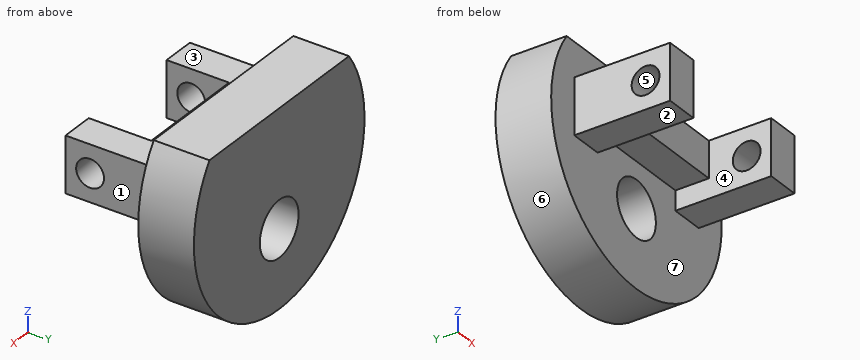
from build123d import *

# Parameters (mm, degrees)
F1_DEPTH = 6.35
F3_D     = 6.35
F2_W     = 3.81
F2_H     = 6.35
F4_DEPTH = 10.9299502
F6_D     = 3.175
F7_W     = 12.7500126
F7_H     = 4.1250048568
F8_DEPTH = 3.81


# Not quite as in the source:
# - a feature names something its author has since deleted; it is built from what else it names


with BuildPart() as f1:
    # F0 (on Front) → F1 (new body)
    with BuildSketch(Plane.XZ):
        with BuildLine():
            Line((11.43, 8.0321852568), (-11.43, 8.0321852568))
            ThreePointArc((-11.43, 8.0321852568), (0, -13.97), (11.43, 8.0321852568))
        make_face()
    extrude(amount=F1_DEPTH)

    # F3 (through all)
    with Locations(Plane.XZ.offset(6.35)):
        with Locations((0, -5.1758147432)):
            Hole(F3_D / 2)

    # F2 (on face) → F4 (join)
    with BuildSketch(Plane.XZ.offset(6.35)):
        with Locations((-8.2800063, 0.9500048568)):
            Rectangle(F2_W, F2_H)
        with Locations((8.2800063, 0.9500048568)):
            Rectangle(F2_W, F2_H)
    extrude(amount=F4_DEPTH)

    # F6 (through all)
    with Locations(Plane(origin=(-10.1850063, 0, 0), x_dir=(0, -1, 0), z_dir=(-1, 0, 0))):
        with Locations((14.478, 0.9500048568)):
            Hole(F6_D / 2)

    # F7 (on face) → F8 (join)
    with BuildSketch(Plane.XZ.offset(6.35)):
        with Locations((0, 2.0625024284)):
            Rectangle(F7_W, F7_H)
    extrude(amount=F8_DEPTH)


solid = f1.part
Part model, mm, in its own coordinate system. Face numbers are marked on the shaded views. A direction names the side the tool comes from. Coordinates: 2 decimals unless noted, no trailing zeros. Loops run counter-clockwise (first coordinate to the right, second up) from the corner with the lowest first, then second, coordinate; pieces in that order, holes last. Notation, with made-up numbers: (-12.5, 18) -> (32.5, 18) arc R22 cw to (32.5, 24) -> close; hole circle Ø10 at (34.25, 19). An arc over 180 degrees is marked (long way). Use a Markdown table: item, result. Add a question column.
Item 1: Band-saw the part on C-C on y = -7.75. Write the cut outline in (x, z) (3 decimals).
Item 2: Probe probe 1 along X at (y, z) = (-14.5, 2.75) (3 decimals); probe 2 along Z at (x, y) = (7.5, -14.5) (3 decimals); probe 3 along Y at (x, z) = (-3, -10.25). List the from-to ranges inside material, lowest first.
Item 3: Flat gauge pins, fed straight in: P1, Ø2, axis at x = -9, y = -3.5, coming from the -Z side; P2, Ø1.9, axis at y = -10, z = 1, coming from the +X side (3 decimals); P3, Ø4, axis at y = -14.48, z = 0.95, coming from the -X side (3 decimals); P4, Ø3.5, axis at x = -3.5, y = -12, coming from the +Z side. Where does each tip first touch, or does it go through?
Item 4: Band-saw the part on B-B on y = -11.75. Write the cut outline in (x, z) (3 decimals).
Item 5: Pull direction Z, two halves, no side cores. Call the marked faces 5, 6 and 7: +Z half, -Z half, draft (parallel to the pull), parting line (faces both ways), or undercut.
Item 6: Which spindle directions (+Z, -Z, +X, -X, +Y, -Y) get a long thin tool onto all of the face, cutting with end or side? Do the marked faces 1, 2, 3 and 4. Say none if no direction does.
Item 7: Band-saw the part on A-A on x = 0. Write the cut outline in (y, z) (3 decimals).
Geometry says:
| question | item | result |
|---|---|---|
| 1 | outline | (-10.185, -2.225) -> (-6.375, -2.225) -> (-6.375, 0) -> (6.375, 0) -> (6.375, -2.225) -> (10.185, -2.225) -> (10.185, 4.125) -> (-10.185, 4.125) -> close |
| 2 | probe 1 | -10.185 to -6.375, 6.375 to 10.185 |
| 2 | probe 2 | -2.225 to -0.637, 2.537 to 4.125 |
| 2 | probe 3 | -6.35 to 0 |
| 3 | P1 | z = -11.45 |
| 3 | P2 | x = 10.185 |
| 3 | P3 | x = -10.185 |
| 3 | P4 | through |
| 4 | outline | (-10.185, -2.225) -> (-6.375, -2.225) -> (-6.375, 4.125) -> (-10.185, 4.125) -> close; (6.375, -2.225) -> (10.185, -2.225) -> (10.185, 4.125) -> (6.375, 4.125) -> close |
| 5 | face 5 | undercut |
| 5 | face 6 | parting line |
| 5 | face 7 | draft |
| 6 | face 1 | +Z, -Z, +X, -Y |
| 6 | face 2 | -Z, +X, -X, -Y |
| 6 | face 3 | +Z, +X, -X, -Y |
| 6 | face 4 | -Z, -Y |
| 7 | outline | (-10.16, 0) -> (-6.35, 0) -> (-6.35, -2.001) -> (0, -2.001) -> (0, 8.032) -> (-6.35, 8.032) -> (-6.35, 4.125) -> (-10.16, 4.125) -> close; (-6.35, -13.97) -> (0, -13.97) -> (0, -8.351) -> (-6.35, -8.351) -> close |
